Geometry check sheet. Reference: drawing and pictorial views, mm from the part's lowest x, y, z. A direction names the side the tool comes from. Round coordinates to 2 decimals unless told otherwise and drop trailing zeros. Write each loop counter-clockwise with the first axis right and the second up, starting at its lowest first coordinate (ties: lowest second). Pieces come first, ordered by that corner, then holes. Notation, with made-up numbers: (16.25, -38) -> (51.25, -38) arc R25 cw to (51.25, -7) -> close; hole circle Ø2 at (62, 85). An arc over 180 degrees is marked (long way). Answer as a JSON object with one key per item and string values. Group by question number.
(1) Sectioned sample at B-B on x = 7.5. Record the cut outline in (y, z).
(2) Sectioned sample at C-C on y = 16. Record the cut outline in (x, z).
(3) Set-up check for the marked faces 4 and 5: record each of +Z, -Z, +X, -X, +Y, -Y from which the full face is reachable in a straight line by a thin tool's end or side.
(4) Sectioned sample at A-A on z = 16. Record the cut outline in (x, y), and give its area (3 significant figures).
(5) Sectioned sample at D-D on x = 33. Record the cut outline in (y, z), and give its area (3 significant figures).
(6) Gauge pin test, flat ends, axial feed: pin 1 Ø6 at (y, z) = (16.5, 15.5) entering from -X; pin 2 Ø3 at (x, y) = (15, 32) entering from -Z; pin 3 Ø5 at (x, y) = (28.5, 34) entering from +Z. Record the tip position at first contact, or that the pin passes through.
(7) Draft check along Z on the marked faces 1, 2 and 3. Enter one of: released by +Z, released by -Z, zero draft, split by the parting line, or undercut.
(8) Scan lines: L1, parallel to Y at x = 6, z = 16; L2, parallel to X at y = 14, z = 13.5; L3, parallel to Z at x = 9.5, y = 36.5. Record each from-to range of solid material in increasing order. Write a range as from..to.
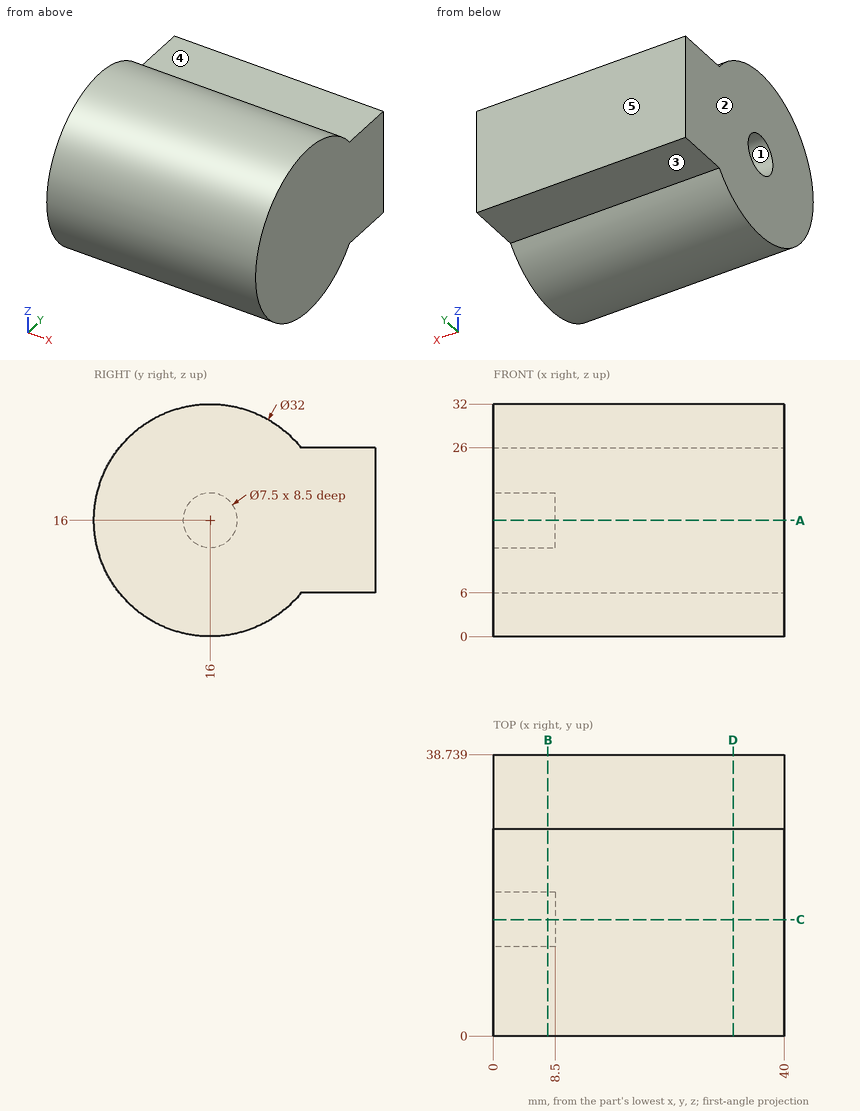
Computed values:
{
 "1": {"outline": "(28.49, 6) -> (38.74, 6) -> (38.74, 26) -> (28.49, 26) arc R16 ccw (long way) to start; hole circle Ø7.5 at (16, 16)"},
 "2": {"outline": "(0, 0) -> (40, 0) -> (40, 32) -> (0, 32) -> (0, 19.75) -> (8.5, 19.75) -> (8.5, 12.25) -> (0, 12.25) -> close"},
 "3": {"face 4": "+Z, +X, -X, +Y", "face 5": "+Z, -Z, +X, -X, +Y"},
 "4": {"outline": "(0, 0) -> (40, 0) -> (40, 38.74) -> (0, 38.74) -> (0, 19.75) -> (8.5, 19.75) -> (8.5, 12.25) -> (0, 12.25) -> close", "area": "1,490 mm2"},
 "5": {"outline": "(28.49, 6) -> (38.74, 6) -> (38.74, 26) -> (28.49, 26) arc R16 ccw (long way) to start", "area": "961 mm2"},
 "6": {"pin 1": "x = 8.5", "pin 2": "z = 6", "pin 3": "z = 26"},
 "7": {"face 1": "undercut", "face 2": "zero draft", "face 3": "released by -Z"},
 "8": {"L1": "0..12.25, 19.75..38.74", "L2": "8.5..40", "L3": "6..26"}
}
